Check sheet for the modelled part. Datum: model origin and axes. Units: mm. A direction names the side the tool comes from. Coordinates: 2 decimals unless noted, no trailing zeros. Write each loop counter-clockwise with the first axis right and the second up, starting at its lowest first coordinate (ties: lowest second). Pieces come first, ordered by that corner, then holes. Notation, with made-up numbers: (81, -30) -> (97, -30) arc R15 cw to (97, -12) -> close; hole circle Ø2 at (-1, 10.5). An arc over 180 degrees is marked (long way). One line per item, written item: value. Start each with the question number.
1) Sectioned sample at A-A on z = 0. Enter the section's corners in (x, y).
2) Sectioned sample at B-B on x = 2.5. Enter the section's corners in (y, z), plus the area to 3 significant figures.
3) Sectioned sample at C-C on y = 2.75. Enter the section's corners in (x, z), plus the area to 3 significant figures.
4) Draft check along X on faces 1 (the cylindrical face through (11.783, 3.631, -0.077)), 2 (the flat face through (1, -2.3, 1)), 3 (the cylindrical face through (0, -4, -1)), 4 (the cylindrical face through (-3.5, 3.6, 0.1)). Enter one of: +X half, -X half, draft (parallel to the pull), parting line (faces both ways), or undercut.
5) Sectioned sample at D-D on x = 8.75. Enter the section's corners in (y, z).
6) Gauge pin test, flat ends, axial feed: P1, Ø1, axis at x = -1.5, y = 0.5, coming from the +Z side; P2, Ø3, axis at y = 0, z = 2, coming from the -X side; P3, Ø3, axis at y = 2.5, z = 1, coming from the -X side. Record the tip position at first contact, or that the pin passes through.
7) Scan lines: line 1 along Z through (x, y) = (0, 4.4); line 2 along Y through (x, z) = (10.75, -2); line 3 along X through (y, z) = (0.25, -0.25). Record each from-to range of solid material in increasing order. Write a range as [from, to].
8) Set-up check for faces 5 (the flat face through (3.292, 0, 0)), 6 (the flat face through (7, -2.3, 0)), 7 (the flat face through (4, 0, -3.5)): record each of +Z, -Z, +X, -X, +Y, -Y from which the full face is reachable in a straight line by a thin tool's end or side.
Autodesk Inventor part; units mm, degrees
ref_plane "YZ Plane" through (0, 0, 0) normal (1, 0, 0) x (0, 1, 0)
ref_plane "XZ Plane" through (0, 0, 0) normal (0, 1, 0) x (-1, 0, 0)
ref_plane "XY Plane" through (0, 0, 0) normal (0, 0, 1) x (1, 0, 0)
sketch "スケッチ1" plane through (0, 0, 0) normal (0, 1, 0) x (-1, 0, 0)
  circle A0 centre (0, 0) radius 1
  circle A1 centre (0, 0) radius 3.5
  circle A2 centre (-8.2843, 0) radius 3.5
  line L0 (0, -3.5) -> (-8.2843, -3.5)
  line L1 (-8.2843, -3.5) -> (-8.2843, 3.5) construction
  line L2 (-8.2843, 3.5) -> (0, 3.5)
  line L3 (0, 3.5) -> (0, -3.5) construction
  circle A3 centre (-8.2843, 0) radius 1
  line L4 (-3.2921, -3.5) -> (-4.9921, -3.5)
  line L5 (-4.9921, -3.5) -> (-4.9921, 3.5)
  line L6 (-4.9921, 3.5) -> (-3.2921, 3.5)
  line L7 (-3.2921, 3.5) -> (-3.2921, -3.5)
  circle A4 centre (-4.1421, 10) radius 10
  line L8 (0, 0) -> (-8.2843, 0)
  line L9 (-4.1421, 10) -> (0, 0)
  line L10 (-4.1421, 10) -> (-8.2843, 0)
  line L11 (-4.1421, -3.5) -> (-4.1421, 3.5) construction
  point P0 (-8.2843, -3.5)
  point P1 (-3.2921, 3.5)
  point P2 (-4.1421, 0)
  dimension "d1" = 7
  dimension "d0" = 2
  dimension "d13" = 20
  dimension "d14" = 45
  dimension "d31" = 1.7
extrude "押し出し3" add sketch "スケッチ1" along normal blind 5 contours A0 A4 A1 L7 L8 | A0 L9 A1 A4 | L8 L7 A4 A0 | A0 A4 L7 A1 L9 | L8 A1 A4 L7 | L7 A1 L8 | L9 L2 A1 | A1 L7 L2 L9 | A4 A1 L7 | L7 L0 L5 A2 L8 A1 | A1 L0 L7 | L8 A4 A1 | A1 A4 A2 L5 L2 L7 | A4 A3 L8 L5 A2 | A2 L10 A3 A4 | L8 A2 A4 | L2 L10 A2 | A2 L5 L0 | A4 L5 A2 | A2 L8 L5 A4 | A2 L5 L8 | L5 A2 L10 L2 | A2 L5 A4 A3 L10 | A3 A4 L5 L8
extrude "押し出し4" cut sketch "スケッチ1" along normal blind 2.3 contours A0 A4 A1 L7 L8 | A0 L9 A1 A4 | L8 L7 A4 A0 | A0 A4 L7 A1 L9 | L9 L2 A1 | A1 L7 L2 L9 | A1 L0 L7 | A4 A3 L8 L5 A2 | A2 L10 A3 A4 | L2 L10 A2 | A2 L5 L0 | L5 A2 L10 L2 | A2 L5 A4 A3 L10 | A3 A4 L5 L8
mirror "ミラー2" about plane through (4.1421, 0, 0) normal (0, -1, 0)
properties part number "chain_1"
Answers:
1. outline: (-3.5, -5) -> (-1, -5) -> (-1, -2.3) -> (-3.5, -2.3) -> close; (-3.5, 2.3) -> (-1, 2.3) -> (-1, 5) -> (-3.5, 5) -> close; (1, -5) -> (7.28, -5) -> (7.28, -2.3) -> (4.99, -2.3) -> (4.99, 2.3) -> (7.28, 2.3) -> (7.28, 5) -> (1, 5) -> (1, 2.3) -> (3.29, 2.3) -> (3.29, -2.3) -> (1, -2.3) -> close; (9.28, -5) -> (11.78, -5) -> (11.78, -2.3) -> (9.28, -2.3) -> close; (9.28, 2.3) -> (11.78, 2.3) -> (11.78, 5) -> (9.28, 5) -> close
2. outline: (-5, -3.5) -> (-2.3, -3.5) -> (-2.3, 3.5) -> (-5, 3.5) -> close; (2.3, -3.5) -> (5, -3.5) -> (5, 3.5) -> (2.3, 3.5) -> close
2. area: 37.8 mm2
3. outline: (0, -3.5) -> (8.28, -3.5) arc R3.5 ccw to (8.28, 3.5) -> (0, 3.5) arc R3.5 ccw to start; hole circle Ø2 at (0, 0); hole circle Ø2 at (8.28, 0)
3. area: 90.2 mm2
4. face 1: +X half
4. face 2: draft
4. face 3: undercut
4. face 4: -X half
5. outline: (-5, -3.47) -> (-2.3, -3.47) -> (-2.3, -0.88) -> (-5, -0.88) -> close; (-5, 0.88) -> (-2.3, 0.88) -> (-2.3, 3.47) -> (-5, 3.47) -> close; (2.3, -3.47) -> (5, -3.47) -> (5, -0.88) -> (2.3, -0.88) -> close; (2.3, 0.88) -> (5, 0.88) -> (5, 3.47) -> (2.3, 3.47) -> close
6. P1: passes through
6. P2: stops at x = 3.29
6. P3: stops at x = -3.5
7. line 1: z = [-3.5, -1], [1, 3.5]
7. line 2: y = [-5, -2.3], [2.3, 5]
7. line 3: x = [3.29, 4.99]
8. face 5: +Z, -Z, -X
8. face 6: +Z, -Z, +X
8. face 7: -Z, +X, -X, +Y, -Y
